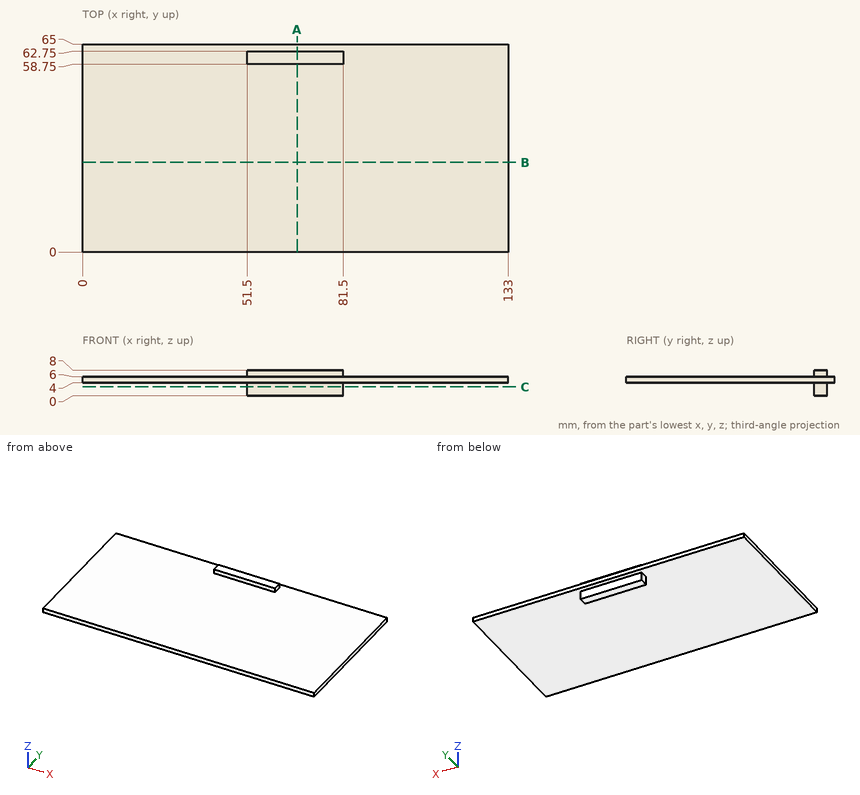
Print and shaded views of the part. All mm, measured from the part's lowest x, y and z. Coordinates: 2 decimals unless noted, no trailing zeros. Write each loop counter-clockwise with the first axis right and the second up, starting at its lowest first coordinate (ties: lowest second). Pieces come first, ordered by that corner, then holes. Notation, with made-up numbers: (25, -26.75) - (58, -26.75) arc R24 cw to (58, 1.25) - close; hole circle Ø11 at (7.5, 64.5). An arc over 180 degrees is marked (long way). One line per question, with ' | ' between items. Start each with the question number.
Q1. Pin check, flat tips, straight feed: pin 1 (0.6 mm diameter, centred on x = 65.5, z = 7, fed in from -Y); pin 2 (2 mm diameter, centred on x = 75, y = 38.5, fed in from -Z); pin 3 (3 mm diameter, centred on y = 61, z = 2, fed in from +X). Stop position of each tip, or through.
Q2. Cut at C-C, the plane z = 2.75. List the corners of the cut face in (x, y), then the cut area to 3 significant figures.
Q3. Cut at A-A, the plane x = 67. List the corners of the cut face in (y, z), then the cut area to 3 significant figures.
Q4. Cut at B-B, the plane y = 28. List the corners of the cut face in (x, z), then the cut area to 3 significant figures.
Q5. Drill centre lines: line 1 (Z direction, x = 34, y = 9.5); line 2 (Y direction, x = 63.5, z = 0.75); line 3 (X direction, y = 62, z = 0.5). Where is each one in solid material? Low to high. Write a range as [from, to].
Answer below:
1) pin 1: y = 58.75 | pin 2: z = 4 | pin 3: x = 81.5
2) outline: (51.5, 58.75) - (81.5, 58.75) - (81.5, 62.75) - (51.5, 62.75) - close | area: 120 mm^2
3) outline: (0, 4) - (58.75, 4) - (58.75, 0) - (62.75, 0) - (62.75, 4) - (65, 4) - (65, 6) - (62.75, 6) - (62.75, 8) - (58.75, 8) - (58.75, 6) - (0, 6) - close | area: 154 mm^2
4) outline: (0, 4) - (133, 4) - (133, 6) - (0, 6) - close | area: 266 mm^2
5) line 1: [4, 6] | line 2: [58.75, 62.75] | line 3: [51.5, 81.5]
